Input: part model. Units: mm. Frame: model coordinates. Face numbers are marked on the shaded views. Coordinates: 2 decimals unless noted, no trailing zeros. Order: outer loops, then holes, each group sorted by start corner. A loop starts at its lowest first (then second) coordinate and runs counter-clockwise, first axis right, second up. Notation, with made-up numbers: (19.25, -24.5) - (76.25, -24.5) arc R18 ccw to (76.25, -5.5) - close; hole circle Ø11 at (52.5, -25.75). An arc over 180 degrees is marked (long way). Answer as CSV lines item,"result". Start each with the question number.
Item 1: First-contact query: pin 1 (2.5 mm diameter, centred on x = 31, y = 19, fed in from -Z); pin 2 (2.5 mm diameter, centred on x = -12.7, y = -20, fed in from +Z); pin 3 (13.5 mm diameter, centred on x = -27.94, y = -19.05, fed in from +Z); pin 4 (9.5 mm diameter, centred on x = 15.24, y = -19.05, fed in from +Z). Flat tips, straight axial feed; report the tip coordinate or a pass-through.
Item 2: Section B-B (z = -1.25). State how many separate pieces and enclosed holes the cut face has, and give its area (3 significant figures).
Item 3: Section D-D (x = -27.94). Output: boundary loops of the cut face in (y, z).
Item 4: Material intervals for line 1 along Y through (x, z) = (31.75, -4.25) (3 decimals); line 2 along X through (y, z) = (-20, 1.5); line 3 along Y through (x, z) = (-9, -2.75), sorted ascending.
Item 5: Section A-A (x = -12.7). Output: boundary loops of the cut face in (y, z) (3 decimals), and give its area (3 significant figures).
Item 6: Draft query along Y for the marked faces 1, 2 and 3. Return one class per face: +Y half, -Y half, draft (parallel to the pull), parting line (faces both ways), or undercut.
from build123d import *

# Parameters (mm, degrees)
F0_W           = 76.2
F0_H           = 76.2
F1_DEPTH       = 6.35
F3_D           = 8.4328
F3_CSINK_D     = 16.6624
F3_CSINK_ANGLE = 82
F5_D           = 4.4
F5_CBORE_D     = 8.25
F5_CBORE_DEPTH = 6.35


with BuildPart() as f1:
    # F0 (on Top) → F1 (new body, symmetric)
    with BuildSketch(Plane.XY):
        Rectangle(F0_W, F0_H)
    extrude(amount=F1_DEPTH, both=True)

    # F3 (through all)
    with Locations(Plane.XY.offset(6.35)):
        with Locations((-27.94, 19.05), (15.24, 19.05), (15.24, -19.05), (-27.94, -19.05)):
            CounterSinkHole(F3_D / 2, F3_CSINK_D / 2, counter_sink_angle=F3_CSINK_ANGLE)

    # F5 (through all)
    with Locations(Plane(origin=(0, 0, -6.35), x_dir=(1, 0, 0), z_dir=(0, 0, -1))):
        with Locations((-12.7, 20), (31.75, 20), (31.75, -20), (-12.7, -20)):
            CounterBoreHole(F5_D / 2, F5_CBORE_D / 2, F5_CBORE_DEPTH)


solid = f1.part
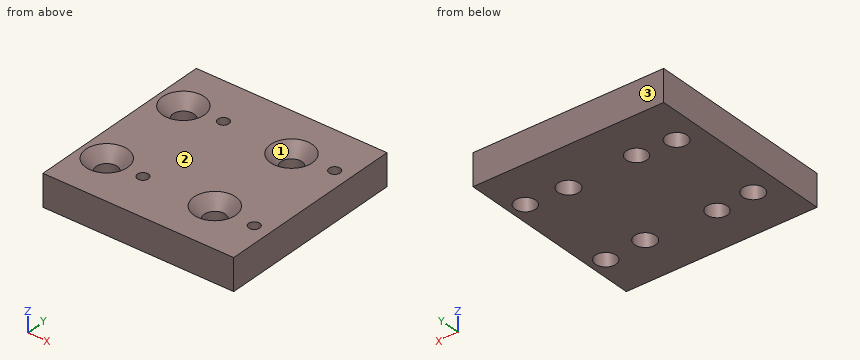
Determined:
1,pin 1,"stops at z = 0"
1,pin 2,"passes through"
1,pin 3,"stops at z = 4.53"
1,pin 4,"stops at z = 2.23"
2,separate pieces,"1"
2,enclosed holes,"8"
2,area,"5,370 mm^2"
3,outline,"(-38.1, -6.35) - (-23.27, -6.35) - (-23.27, 1.62) - (-27.38, 6.35) - (-38.1, 6.35) - close; (-14.83, -6.35) - (14.83, -6.35) - (14.83, 1.62) - (10.72, 6.35) - (-10.72, 6.35) - (-14.83, 1.62) - close; (23.27, -6.35) - (38.1, -6.35) - (38.1, 6.35) - (27.38, 6.35) - (23.27, 1.62) - close"
4,line 1,"y = -38.1 to -24.125, -15.875 to 15.875, 24.125 to 38.1"
4,line 2,"x = -38.1 to -32.05, -23.83 to -14.9, -10.5 to 11.13, 19.35 to 29.55, 33.95 to 38.1"
4,line 3,"y = -38.1 to -21.82, -18.18 to 18.18, 21.82 to 38.1"
5,outline,"(-38.1, -6.35) - (-24.125, -6.35) - (-24.125, 0) - (-22.2, 0) - (-22.2, 6.35) - (-38.1, 6.35) - close; (-17.8, 0) - (-15.875, 0) - (-15.875, -6.35) - (15.875, -6.35) - (15.875, 0) - (17.8, 0) - (17.8, 6.35) - (-17.8, 6.35) - close; (22.2, 0) - (24.125, 0) - (24.125, -6.35) - (38.1, -6.35) - (38.1, 6.35) - (22.2, 6.35) - close"
5,area,"807 mm^2"
6,face 1,"undercut"
6,face 2,"draft"
6,face 3,"+Y half"
